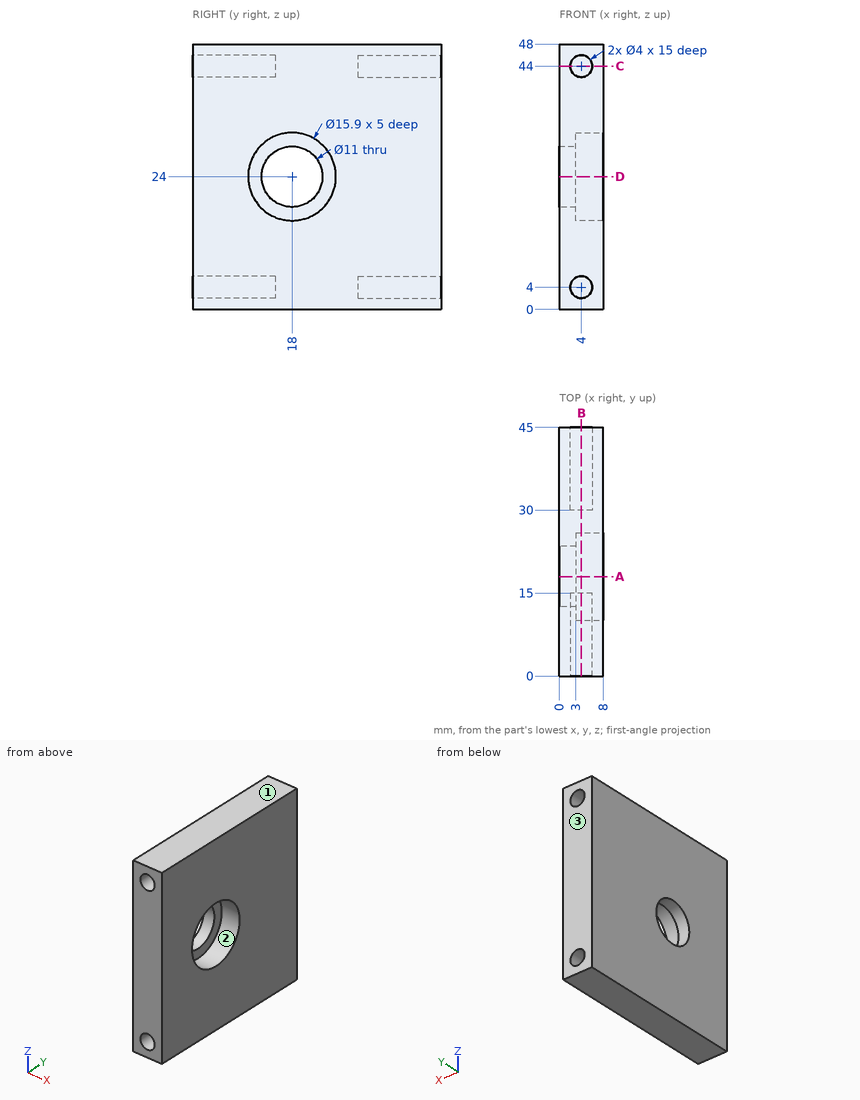
Here's the drawing with two shaded views (mm, measured from the low corner). I have some questions. Coordinates: 2 decimals unless noted, no trailing zeros. Loops run counter-clockwise (first coordinate to the right, second up) from the corner with the lowest first, then second, coordinate; pieces in that order, holes last. Notation, with made-up numbers: (-19, 37.5) - (13, 37.5) arc R18 cw to (13, 44.5) - close; hole circle Ø4 at (10, 26.5). An arc over 180 degrees is marked (long way). Answer as CSV lines item,"result". Start each with the question number.
1) I need wall thicknesses on line 1 (Z direction, x = 4, y = 35.75); line 2 (Y direction, x = 0.9, z = 24); line 3 (X direction, y = 41, z = 44). Which ranges of each line are inside material? Lowest first, please. Write a range as from..to.
2) Suppose I cut it at D-D (z = 24). Please give me the cut outline in (x, y), plus the area to 4 significant figures.
3) For pin 1 (12.5 mm diameter, centred on y = 18, z = 24, fed in from +X); pin 2 (3.5 mm diameter, centred on x = 4, z = 44, fed in from -Y), each with a flat end and sliding along its axis, tell me the tip position at first contact or that it passes through.
4) Thinking about a two-plate mould opening in Y: for the marked faces 1, 2 and 3, which applies, pulls with the +Y half, pulls with the -Y half, needs draft (parallel to the pull), parting line crosses it, or undercut?
5) Suppose I cut it at B-B (x = 4). Please give me the cut outline in (y, z), plus the area to 3 significant figures.
6) Suppose I cut it at A-A (y = 18). Please give me the cut outline in (x, z).
7) Suppose I cut it at C-C (z = 44). Please give me the cut outline in (x, y).
Check result:
1,line 1,"z = 0..2, 6..42, 46..48"
1,line 2,"y = 0..12.5, 23.5..45"
1,line 3,"x = 0..2, 6..8"
2,outline,"(0, 0) - (8, 0) - (8, 10.05) - (3, 10.05) - (3, 12.5) - (0, 12.5) - close; (0, 23.5) - (3, 23.5) - (3, 25.95) - (8, 25.95) - (8, 45) - (0, 45) - close"
2,area,"247.5 mm²"
3,pin 1,"stops at x = 3"
3,pin 2,"stops at y = 15"
4,face 1,"needs draft"
4,face 2,"undercut"
4,face 3,"pulls with the +Y half"
5,outline,"(0, 0) - (45, 0) - (45, 2) - (30, 2) - (30, 6) - (45, 6) - (45, 42) - (30, 42) - (30, 46) - (45, 46) - (45, 48) - (0, 48) - (0, 46) - (15, 46) - (15, 42) - (0, 42) - (0, 6) - (15, 6) - (15, 2) - (0, 2) - close; hole circle Ø15.9 at (18, 24)"
5,area,"1,720 mm²"
6,outline,"(0, 0) - (8, 0) - (8, 16.05) - (3, 16.05) - (3, 18.5) - (0, 18.5) - close; (0, 29.5) - (3, 29.5) - (3, 31.95) - (8, 31.95) - (8, 48) - (0, 48) - close"
7,outline,"(0, 0) - (2, 0) - (2, 15) - (6, 15) - (6, 0) - (8, 0) - (8, 45) - (6, 45) - (6, 30) - (2, 30) - (2, 45) - (0, 45) - close"
